Verification items for the finished model (mm, model axes). A direction names the side the tool comes from. Coordinates: 2 decimals unless noted, no trailing zeros. Write each loop counter-clockwise with the first axis right and the second up, starting at its lowest first coordinate (ties: lowest second). Pieces come first, ordered by that corner, then holes. Notation, with made-up numbers: (27, -27.5) -> (35, -27.5) arc R23 cw to (35, -9.5) -> close; hole circle Ø6 at (82, 26.5). An arc over 180 degrees is marked (long way). Answer in a Markdown table with one row per item.
```python
from build123d import *

# Parameters (mm, degrees)
BOSS_EXTRUDE1_DEPTH     = 35
CUT_EXTRUDE1_DEPTH      = 165.23458831805192
CUT_EXTRUDE1_DEPTH_BACK = 165.23458831805192
CUT_EXTRUDE2_DEPTH      = 165.23458831805192
CUT_EXTRUDE3_DEPTH      = 165.23458831805192
CUT_EXTRUDE4_REACH      = 166.235
SKETCH7_R               = 4.1
SKETCH7_R_2             = 4.099999999999986
SKETCH7_3_R             = 11.1
CUT_EXTRUDE5_DEPTH      = 7.1
FILLET1_R               = 9
FILLET2_START           = 9
FILLET2_DEPTH           = 26


with BuildPart() as part:
    # Sketch1 → Boss-Extrude1 (new body)
    with BuildSketch(Plane(origin=(0, 0, 0), x_dir=(0, 0, -1), z_dir=(1, 0, 0))):
        with BuildLine():
            ThreePointArc((-3.4331525583588727, 27.788729073331762), (-20.97770568525129, 18.545507924642443), (-28, 3.43e-15))
            Line((-28, 0), (28, 0))
            ThreePointArc((28, 0), (18.545507924642447, 20.977705685251287), (-3.4331525583588727, 27.788729073331762))
        make_face()
        with BuildLine():
            Line((28, 0), (-28, 0))
            ThreePointArc((-28, 3.43e-15), (-20.977705685251298, -18.545507924642436), (-3.433152558358892, -27.78872907333176))
            ThreePointArc((-3.433152558358892, -27.78872907333176), (18.545507924642436, -20.977705685251298), (28, -6.86e-15))
        make_face()
        with BuildLine():
            ThreePointArc((-126.56684744164114, 27.788729073331766), (-109.02229431474872, 18.54550792464245), (-102, 0))
            Line((-102, 0), (-28, 0))
            ThreePointArc((-28, 3.43e-15), (-20.97770568525129, 18.545507924642443), (-3.4331525583588727, 27.788729073331762))
            ThreePointArc((-3.433152558358863, 27.788729073331695), (-65, 23.999999999999602), (-126.56684744164116, 27.788729073331638))
        make_face()
        with BuildLine():
            Line((-28, 0), (-102, 0))
            ThreePointArc((-102, -6.86e-15), (-109.0222943147487, -18.545507924642447), (-126.56684744164114, -27.788729073331766))
            ThreePointArc((-126.56684744164116, -27.788729073331638), (-65, -23.999999999999602), (-3.433152558358863, -27.788729073331695))
            ThreePointArc((-3.433152558358892, -27.78872907333176), (-20.977705685251298, -18.545507924642436), (-28, 3.43e-15))
        make_face()
        with BuildLine():
            ThreePointArc((-126.56684744164114, 27.788729073331766), (-148.54550792464244, 20.977705685251287), (-158, 3.43e-15))
            Line((-158, 0), (-102, 0))
            ThreePointArc((-102, 0), (-109.02229431474872, 18.54550792464245), (-126.56684744164114, 27.788729073331766))
        make_face()
        with BuildLine():
            Line((-102, 0), (-158, 0))
            ThreePointArc((-158, 3.43e-15), (-148.54550792464244, -20.97770568525128), (-126.56684744164114, -27.788729073331766))
            ThreePointArc((-126.56684744164114, -27.788729073331766), (-109.0222943147487, -18.545507924642447), (-102, -6.86e-15))
        make_face()
    extrude(amount=BOSS_EXTRUDE1_DEPTH)

    # Sketch4 → Cut-Extrude1 (cut, two sides: drawn at the far end of the back side and taken through both)
    with BuildSketch(Plane(origin=(0, 0, 0), x_dir=(1, 0, 0), z_dir=(0, 1, 0)).offset(-CUT_EXTRUDE1_DEPTH_BACK)):
        Polygon((8.999999999999998, 27.999999999999996), (61, 27.999999999999996), (61, -28.000000000000004), (9.000000000000005, -28.000000000000004), align=None)
        Polygon((60.999999999999986, -157.99999999999997), (60.99999999999993, -101.99999999999999), (8.999999999999956, -101.99999999999999), (8.99999999999997, -157.99999999999997), align=None)
    extrude(amount=CUT_EXTRUDE1_DEPTH + CUT_EXTRUDE1_DEPTH_BACK, mode=Mode.SUBTRACT)

    # Sketch6 → Cut-Extrude2 (cut, through all)
    with BuildSketch(Plane(origin=(0, 0, 0), x_dir=(0, 0, -1), z_dir=(1, 0, 0))):
        with BuildLine():
            Line((-30.624999999999996, -21.1), (-66.82499999999999, -21.100000000000005))
            ThreePointArc((-66.82499999999999, -21.100000000000005), (-68.94632034355963, -20.221320343559647), (-69.825, -18.100000000000005))
            Line((-69.825, -18.100000000000005), (-69.825, 18.099999999999998))
            ThreePointArc((-69.825, 18.099999999999998), (-68.94632034355963, 20.22132034355964), (-66.82499999999999, 21.099999999999998))
            Line((-66.82499999999999, 21.099999999999998), (-30.624999999999996, 21.1))
            ThreePointArc((-30.624999999999996, 21.1), (-28.503679656440355, 20.221320343559643), (-27.624999999999996, 18.1))
            Line((-27.624999999999996, 18.1), (-27.624999999999996, -18.1))
            ThreePointArc((-27.624999999999996, -18.1), (-28.503679656440355, -20.221320343559643), (-30.624999999999996, -21.1))
        make_face()
    extrude(amount=CUT_EXTRUDE2_DEPTH, mode=Mode.SUBTRACT)

    # Sketch8 → Cut-Extrude3 (cut, through all)
    with BuildSketch(Plane(origin=(0, 0, 0), x_dir=(0, 0, -1), z_dir=(1, 0, 0))):
        Polygon((-99.99999999999986, 15.499999999999991), (-96.9999999999999, 10.303847577293476), (-91.00000000000006, 10.303847577293476), (-88.00000000000014, 15.500000000000032), (-91.00000000000013, 20.696152422706533), (-96.99999999999999, 20.69615242270647), align=None)
        Polygon((-99.99521646144645, -15.739540352344857), (-96.7901602003611, -20.811779932971724), (-90.79494373891465, -20.57223958062687), (-88.00478353855354, -15.26045964765515), (-91.20983979963889, -10.188220067028302), (-97.20505626108536, -10.427760419373156), align=None)
    extrude(amount=CUT_EXTRUDE3_DEPTH, mode=Mode.SUBTRACT)

    # Sketch7 → Cut-Extrude4 (cut, up to next)
    with BuildSketch(Plane(origin=(0, 0, 0), x_dir=(0, 0, -1), z_dir=(1, 0, 0)), mode=Mode.PRIVATE) as cut_extrude4_sk1:
        with Locations(Location((0, 0, 0), (0, 0, 180))):
            Circle(SKETCH7_R)
    cut_extrude4_tool1 = extrude(cut_extrude4_sk1.sketch, amount=CUT_EXTRUDE4_REACH, mode=Mode.PRIVATE) & part.part
    # Sketch7 → Cut-Extrude4 (cut, up to next)
    with BuildSketch(Plane(origin=(0, 0, 0), x_dir=(0, 0, -1), z_dir=(1, 0, 0)), mode=Mode.PRIVATE) as cut_extrude4_sk2:
        with Locations(Location((-130, 0, 0), (0, 0, 180))):
            Circle(SKETCH7_R_2)
    cut_extrude4_tool2 = extrude(cut_extrude4_sk2.sketch, amount=CUT_EXTRUDE4_REACH, mode=Mode.PRIVATE) & part.part
    add(cut_extrude4_tool1.solids().sort_by_distance((0, 0, 0))[0], mode=Mode.SUBTRACT)
    add(cut_extrude4_tool2.solids().sort_by_distance((0, 0, 130))[0], mode=Mode.SUBTRACT)

    # Sketch7<3> → Cut-Extrude5 (cut)
    with BuildSketch(Plane(origin=(0, 0, 0), x_dir=(0, 0, -1), z_dir=(1, 0, 0))):
        Circle(SKETCH7_3_R)
        with Locations((-130, 0)):
            Circle(SKETCH7_3_R)
    extrude(amount=CUT_EXTRUDE5_DEPTH, mode=Mode.SUBTRACT)

    # Fillet1
    # the kernel refuses this fillet: 9 mm, written as the material it takes off along each edge
    with BuildSketch(Plane(origin=(0, -7.11e-15, 130), x_dir=(0, 0.9924546097618487, -0.12261259136995861), z_dir=(0, -0.12261259136995861, -0.9924546097618487))) as fillet1_piece_1:
        with BuildLine():
            CenterArc((28 - FILLET1_R, FILLET1_R), FILLET1_R, 270, 89.99999999999999)
            Line((28, FILLET1_R), (28, 0))
            Line((28, 0), (28 - FILLET1_R, 0))
        make_face()
    revolve(axis=Axis((0, -7.11e-15, 130), (1, 0, 0)), revolution_arc=194.0858135076888, mode=Mode.SUBTRACT)
    with BuildSketch(Plane(origin=(0, 526.1249999999663, 65.00000000000024), x_dir=(0, -0.9924546097618476, -0.12261259136996856), z_dir=(0, 0.12261259136996856, -0.9924546097618476))) as fillet1_piece_2:
        with BuildLine():
            CenterArc((502.12499999996675 + FILLET1_R, -FILLET1_R), FILLET1_R, 90, 90)
            Line((502.12499999996675 + FILLET1_R, 1.78e-15), (502.12499999996675, 0))
            Line((502.12499999996675, 0), (502.12499999996675, -FILLET1_R))
        make_face()
    revolve(axis=Axis((0, 526.1249999999663, 65.00000000000024), (-1, 0, 0)), revolution_arc=14.085813507689899, mode=Mode.SUBTRACT)
    with BuildSketch(Plane(origin=(0, 1.78e-15, -1.78e-15), x_dir=(0, -0.9924546097618486, 0.12261259136995943), z_dir=(0, 0.12261259136995943, 0.9924546097618486))) as fillet1_piece_3:
        with BuildLine():
            CenterArc((28 - FILLET1_R, FILLET1_R), FILLET1_R, 270, 90)
            Line((27.999999999999996, FILLET1_R), (28, 0))
            Line((28, 0), (28 - FILLET1_R, 0))
        make_face()
    revolve(axis=Axis((0, 1.78e-15, -1.78e-15), (1, 0, 0)), revolution_arc=194.0858135076889, mode=Mode.SUBTRACT)
    with BuildSketch(Plane(origin=(0, -526.1249999999588, 65.00000000000026), x_dir=(0, 0.9924546097618475, 0.12261259136996942), z_dir=(0, -0.12261259136996942, 0.9924546097618475))) as fillet1_piece_4:
        with BuildLine():
            CenterArc((502.1249999999594 + FILLET1_R, -FILLET1_R), FILLET1_R, 90, 90)
            Line((502.1249999999594 + FILLET1_R, 1.78e-15), (502.1249999999594, 0))
            Line((502.1249999999594, 0), (502.1249999999594, -FILLET1_R))
        make_face()
    revolve(axis=Axis((0, -526.1249999999588, 65.00000000000026), (-1, 0, 0)), revolution_arc=14.085813507690109, mode=Mode.SUBTRACT)

    # Fillet2: read off the stored shape, not the designer's step
    # Fillet2 outline → Fillet2 (cut)
    with BuildSketch(Plane.YZ.offset(FILLET2_START)):
        with BuildLine():
            ThreePointArc((25.365061881, 28), (25.062921918, 32.34560469), (24.798492486, 36.693666988))
            ThreePointArc((24.798492486, 36.693666988), (23.518514891, 31.536360045), (19.552368755, 28))
            Line((19.552368755, 28), (25.365061881, 28))
        make_face()
        with BuildLine():
            Line((25.365061881, 102), (15.767511934, 102))
            ThreePointArc((15.767511934, 102), (22.303461396, 99.187193599), (24.753997417, 92.506969919))
            ThreePointArc((24.753997417, 92.506969919), (25.037048655, 97.254932057), (25.365061881, 102))
        make_face()
        with BuildLine():
            ThreePointArc((-25.365061881, 102), (-25.037048655, 97.254932057), (-24.753997417, 92.506969919))
            ThreePointArc((-24.753997417, 92.506969919), (-22.303461396, 99.187193599), (-15.767511934, 102))
            Line((-15.767511934, 102), (-25.365061881, 102))
        make_face()
        with BuildLine():
            ThreePointArc((-19.552368755, 28), (-23.518514891, 31.536360045), (-24.798492486, 36.693666988))
            ThreePointArc((-24.798492486, 36.693666988), (-25.062921918, 32.34560469), (-25.365061881, 28))
            Line((-25.365061881, 28), (-19.552368755, 28))
        make_face()
    extrude(amount=FILLET2_DEPTH, mode=Mode.SUBTRACT)


solid = part.part
```
1. Material ranges on probe 1 along Z at (x, y) = (8, 20); probe 2 along X at (y, z) = (21.5, 104); probe 3 along X at (y, z) = (-6, -10), recorded low to high. Write a range as from..to.
Findings below:
| item | result |
|---|---|
| probe 1 | z = -19.52..28.3, 69.15..90.6, 97.4..149.52 |
| probe 2 | x = 1.51..9 |
| probe 3 | x = 0..9 |
2. Go/stop test with flat-tipped pins: pin 1 (4 mm diameter, centred on x = 20.5, z = 83, fed in from -Y); pin 2 (8 mm diameter, centred on x = 15, y = 0.5, fed in from -Z) (3 decimals); pin 3 (10 mm diameter, centred on x = 19, y = -18, fed in from +Z). Record where each tip stops, or that it passes through.
Findings below:
| item | result |
|---|---|
| pin 1 | stops at y = -24.4 |
| pin 2 | stops at z = 69.825 |
| pin 3 | stops at z = 102 |
3. Release check for a two-part mould opening along Z. For faces 1 (the face through (17.34, -20.54, 28.88)), 2 (the face through (35, 0, 74)) record: released by +Z, released by -Z, zero draft, split by the parting line, or undercut.
Findings below:
| item | result |
|---|---|
| face 1 | undercut |
| face 2 | zero draft |
4. Sectioned sample at C-C, the plane z = 130. Record the cut outline in (x, y), and give its area (3 significant figures).
Findings below:
| item | result |
|---|---|
| outline | (0, -19) arc R9 ccw to (9, -28) -> (9, -4.1) -> (7.1, -4.1) -> (7.1, -11.1) -> (0, -11.1) -> close; (0, 11.1) -> (7.1, 11.1) -> (7.1, 4.1) -> (9, 4.1) -> (9, 28) arc R9 ccw to (0, 19) -> close |
| area | 296 mm² |
5. Sectioned sample at B-B, the plane x = 29.5. Count the separate pieces of the cut face and the enclosed holes in it, and give its area (3 significant figures).
Findings below:
| item | result |
|---|---|
| separate pieces | 1 |
| enclosed holes | 2 |
| area | 1,600 mm² |
6. Access from +Z, -Z, +X, -X, +Y, -Y to the whole of each face (thin tool, end or side, straight path). Record for faces 3 (the face through (18, 20.696, 94)), 4 (the face through (7.1, 0, -5)), 5 (the face through (0, 0, 15)).
Findings below:
| item | result |
|---|---|
| face 3 | +X, -X |
| face 4 | -X |
| face 5 | +Z, -Z, -X, +Y, -Y |
7. Sectioned sample at A-A, the plane y = 0. Record the cut outline in (x, z) (3 decimals).
Findings below:
| item | result |
|---|---|
| outline | (0, -19) arc R9 ccw to (9, -28) -> (9, -4.1) -> (7.1, -4.1) -> (7.1, -11.1) -> (0, -11.1) -> close; (0, 11.1) -> (7.1, 11.1) -> (7.1, 4.1) -> (9, 4.1) -> (9, 27.625) -> (0, 27.625) -> close; (0, 69.825) -> (35, 69.825) -> (35, 102) -> (9, 102) -> (9, 125.9) -> (7.1, 125.9) -> (7.1, 118.9) -> (0, 118.9) -> close; (0, 141.1) -> (7.1, 141.1) -> (7.1, 134.1) -> (9, 134.1) -> (9, 158) arc R9 ccw to (0, 149) -> close |
